from build123d import *

# Parameters (mm, degrees)
F1_DEPTH = 40
F2_R     = 5
F3_R     = 5


with BuildPart() as f1:
    # F0 (on Front) → F1 (new body)
    with BuildSketch(Plane.XZ):
        Polygon((-49.333352, 37.356967), (-69.333352, 37.356967), (-69.333352, -12.643033), (48.288023, -12.643033), (48.288023, 37.356967), (28.288023, 37.356967), (0, 0), align=None)
    extrude(amount=F1_DEPTH)

    # F2
    f2_edges = [f1.edges().sort_by_distance(p)[0] for p in [
        (0, -20, 0),
    ]]
    fillet(f2_edges, radius=F2_R)

    # F3
    f3_edges = [f1.edges().sort_by_distance(p)[0] for p in [
        (-69.333352, -20, 37.356967),
        (48.288023, -20, 37.356967),
        (-49.333352, -20, 37.356967),
        (28.288023, -20, 37.356967),
    ]]
    fillet(f3_edges, radius=F3_R)


solid = f1.part
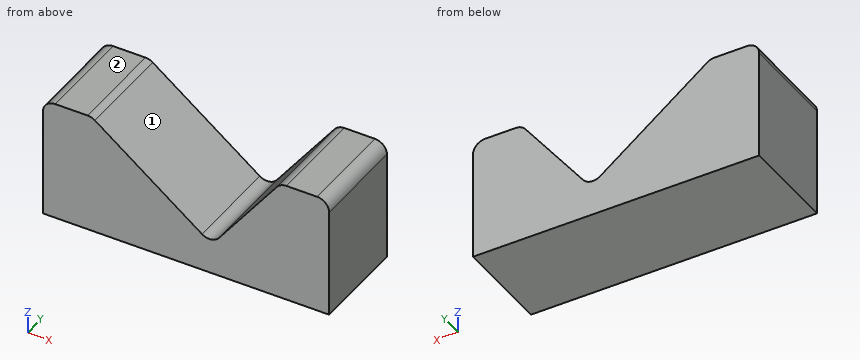
CAD build for the part. Positions are in the model's coordinates, mm. Face numbers are marked on the shaded views. A direction names the side the tool comes from. Give positions to 0.01 mm unless a question says otherwise; leave off trailing zeros. Order: outer loops, then holes, each group sorted by start corner. A loop starts at its lowest first (then second) coordinate and runs counter-clockwise, first axis right, second up. Notation, with made-up numbers: (-33, -38.5) -> (-7, -38.5) arc R21 ccw to (-7, -15.5) -> close; hole circle Ø8 at (50, 44.25). An arc over 180 degrees is marked (long way). Return JSON: item names as keys, results as strings.
Q1. Saw through at B-B (y = -9). Write the cut outline in (x, z).
Working result:
{"outline": "(-69.33, -12.64) -> (48.29, -12.64) -> (48.29, 32.36) arc R5 ccw to (43.29, 37.36) -> (30.77, 37.36) arc R5 ccw to (26.79, 35.38) -> (3.02, 3.99) arc R5 cw to (-3.99, 3.02) -> (-47.99, 36.34) arc R5 ccw to (-51.01, 37.36) -> (-64.33, 37.36) arc R5 ccw to (-69.33, 32.36) -> close"}
Q2. Drill centre lines: line 1 (X direction, y = -32, z = 8); line 2 (X direction, y = -34, z = 20); line 3 (Z direction, x = 22.5, y = -30.5). Where is each one in solid material? Low to high.
Working result:
{"line 1": "-69.33 to -10.56, 6.06 to 48.29", "line 2": "-69.33 to -26.41, 15.14 to 48.29", "line 3": "-12.64 to 29.71"}
Q3. Which spindle directions (+Z, -Z, +X, -X, +Y, -Y) get a long thin tool onto all of the face, cutting with end or side? Do the marked faces 1 and 2. Say none if no direction does.
Working result:
{"face 1": "+Z, +Y, -Y", "face 2": "+Z, +X, -X, +Y, -Y"}
Q4. Saw through at D-D (x = -40.5). Write the cut outline in (y, z).
Working result:
{"outline": "(-40, -12.64) -> (0, -12.64) -> (0, 30.67) -> (-40, 30.67) -> close"}
Q5. Saw through at C-C (z = 16). Write the cut outline in (x, y), then the cut area to 3 significant figures.
Working result:
{"outline": "(-69.33, -40) -> (-21.13, -40) -> (-21.13, 0) -> (-69.33, 0) -> close; (12.12, -40) -> (48.29, -40) -> (48.29, 0) -> (12.12, 0) -> close", "area": "3,380 mm²"}
Q6. Saw through at A-A (z = 8). Write the cut outline in (x, y), then the cut area to 3 significant figures.
Working result:
{"outline": "(-69.33, -40) -> (-10.56, -40) -> (-10.56, 0) -> (-69.33, 0) -> close; (6.06, -40) -> (48.29, -40) -> (48.29, 0) -> (6.06, 0) -> close", "area": "4,040 mm²"}
